The listing builds one solid part. Answer for the finished solid, in the listing's coordinates (mm). A direction names the side the tool comes from. Round coordinates to 2 decimals unless told otherwise and drop trailing zeros. One line per question, with ' | ' between items. Start each with the question number.
from build123d import *

# Parameters (mm, degrees)
EXTRUDE_THIN1_DEPTH = 412.75
FILLET1_R           = 1.27


with BuildPart() as part:
    # Sketch1 → Extrude-Thin1 (new body)
    with BuildSketch(Plane.XY):
        with BuildLine():
            Line((0, 41.275), (-14.2875, 41.275))
            Line((-14.2875, 41.275), (-14.2875, 32.940625))
            Line((-14.2875, 32.940625), (-11.90625, 32.940625))
            Line((-11.90625, 32.940625), (-11.90625, 29.765625))
            ThreePointArc((-11.90625, 29.765625), (-7.793372209, 25.995204752), (-5.693451363, 20.825856146))
            ThreePointArc((-5.693451363, 20.825856146), (-4.995631362, 15.194568327), (-4.7625, 9.525))
            Line((-4.7625, 9.525), (-6.35, 9.525))
            ThreePointArc((-6.35, 9.525), (-9.525, 6.35), (-6.35, 3.175))
            Line((-6.35, 3.175), (-4.7625, 3.175))
            Line((-4.7625, 3.175), (-4.7625, 0))
            Line((-4.7625, 0), (0, 0))
            Line((0, 0), (0, 1.27))
            Line((0, 1.27), (-3.4925, 1.27))
            Line((-3.4925, 1.27), (-3.4925, 4.445))
            Line((-3.4925, 4.445), (-6.35, 4.445))
            ThreePointArc((-6.35, 4.445), (-8.255, 6.35), (-6.35, 8.255))
            Line((-6.35, 8.255), (-3.503968204, 8.255))
            ThreePointArc((-3.503968204, 8.255), (-3.680640178, 14.665718794), (-4.440572307, 21.033687983))
            ThreePointArc((-4.440572307, 21.033687983), (-6.541275078, 26.410168765), (-10.63625, 30.47842123))
            Line((-10.63625, 30.47842123), (-10.63625, 34.210625))
            Line((-10.63625, 34.210625), (-13.0175, 34.210625))
            Line((-13.0175, 34.210625), (-13.0175, 40.005))
            Line((-13.0175, 40.005), (0, 40.005))
            Line((0, 40.005), (0, 41.275))
        make_face()
    extrude(amount=-EXTRUDE_THIN1_DEPTH)

    # Fillet1
    fillet1_edges = [part.edges().sort_by_distance(p)[0] for p in [
        (-4.7625, 0, -206.375),
        (-11.90625, 29.765625, -206.375),
        (-14.2875, 32.940625, -206.375),
        (-14.2875, 41.275, -206.375),
        (-10.63625, 34.210625, -206.375),
        (-3.503968204, 8.255, -206.375),
        (-3.4925, 4.445, -206.375),
    ]]
    fillet(fillet1_edges, radius=FILLET1_R)


solid = part.part
(1) Determine the mould class of faces 4 (the cylindrical face through (-7.644, 25.775, -203.486)), 5 (the flat face through (-6, 41.275, -203)), 6 (the flat face through (-6, 24, 0)) for opening direction Y: pulls with the +Y half, pulls with the -Y half, needs draft (parallel to the pull), parting line crosses it, or undercut.
(2) Each of these flat-tipped pins is pushed along its axis until it touches: P1, Ø6, axis at y = 13.5, z = -110, coming from the -X side; P2, Ø0.8, axis at x = -5.5, z = -172.5, coming from the -Y side (3 decimals); P3, Ø12, axis at y = 20, z = -74, coming from the -X side. Where does it stop, or does it pass through?
(3) A tool of negligible diameter and unlimited length cuts with its end or side. For faces 1 (the flat face through (-6, 24, -412.75)), 2 (the cylindrical face through (-6.497, 26.342, -203.486)), 3 (the cylindrical face through (-5, 15.27, -203.49)), from which of +Z, -Z, +X, -X, +Y, -Y can it reach the whole face along a straight path? Write none if from no direction.
(4) Consider L1, parallel to Y at x = -1.5, z = -283.5 (3 decimals); L2, parallel to Y at x = -12.5, z = -300 (3 decimals); L3, parallel to X at y = 2, z = -152. Determine where each line is inside the solid, lowest interval first.
Answer below:
1) face 4: undercut | face 5: pulls with the +Y half | face 6: needs draft
2) P1: x = -5.12 | P2: y = 3.175 | P3: x = -7.8
3) face 1: -Z, +X, -X, +Y, -Y | face 2: +Z, -Z, +X | face 3: +Z, -Z, -X
4) L1: 0 to 1.27, 40.005 to 41.275 | L2: 32.941 to 34.211, 40.005 to 41.275 | L3: -4.76 to -3.49
